Could you check a few things on this drawing? It's one solid part, dimensions in mm from its lowest x, y, z. A direction names the side the tool comes from. Coordinates: 2 decimals unless noted, no trailing zeros. Loops run counter-clockwise (first coordinate to the right, second up) from the corner with the lowest first, then second, coordinate; pieces in that order, holes last.
1) For the marked faces 4 and 5, which set-ups out of +Z, -Z, +X, -X, +Y, -Y let a thin tool reach every point of the face, with its end or its side?
2) Imagine slicing it at D-D on z = 17. Please give me the cut outline in (x, y).
3) Thinking about a two-plate mould opening in Y: for the marked faces 1, 2 and 3, which applies, released by +Y, released by -Y, zero draft, split by the parting line, or undercut?
4) Imagine slicing it at C-C on x = 11. Give the number of separate pieces and of enclosed holes in the cut face.
5) Will these pins go through, and if not, where does the flat tip stop? P1, Ø1, axis at x = 33.5, z = 22.5, coming from the -Y side; P2, Ø5, axis at x = 6.35, y = 51.66, coming from the -Z side; P3, Ø4, axis at x = 11.575, z = 9.525, coming from the +Y side; P4, Ø2, axis at x = 6.5, z = 43.5, coming from the +Y side.
6) If I drill on line 1 along Y through (x, z) = (15, 21); line 2 along Z through (x, y) = (53.5, 46.5); line 3 along Y through (x, z) = (6, 60) (1 decimal), over which ranges is the centre line in solid material (lowest first)?
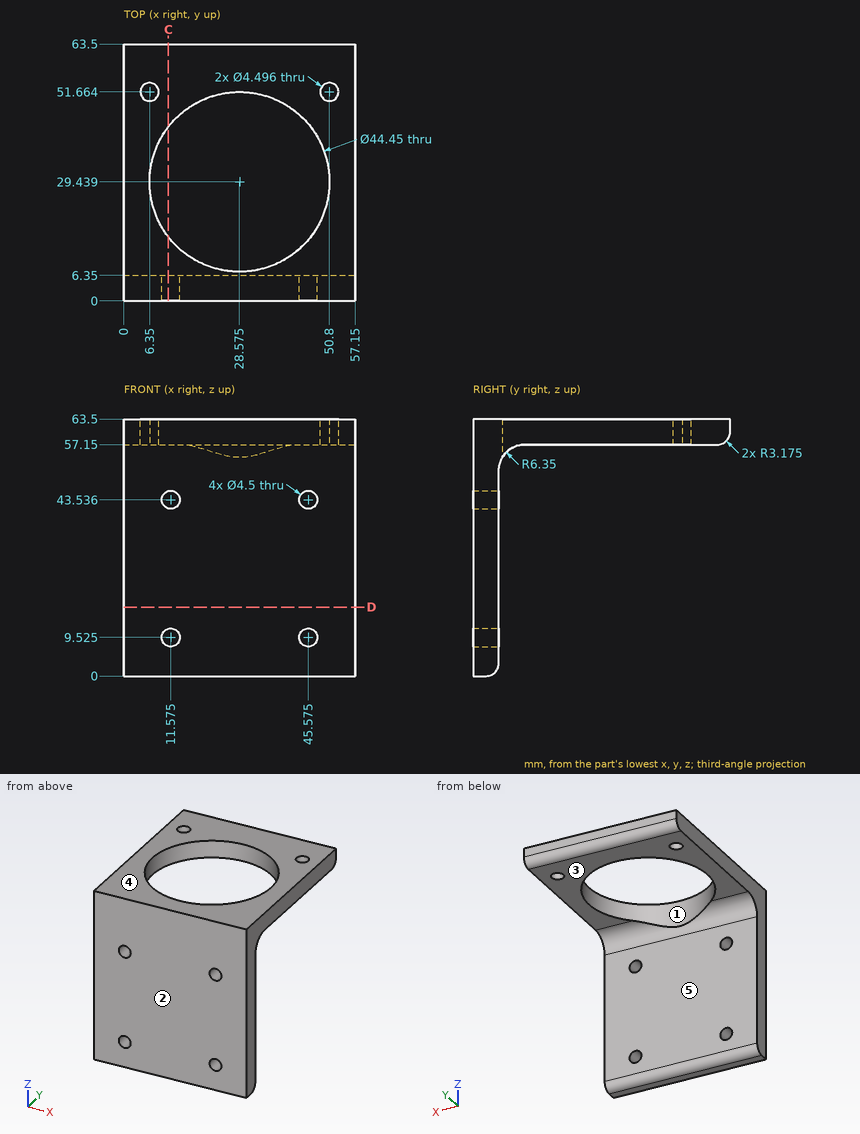
Filled in:
1. face 4: +Z, +X, -X, +Y, -Y
1. face 5: -Z, +X, -X, +Y
2. outline: (0, 0) - (57.15, 0) - (57.15, 6.35) - (0, 6.35) - close
3. face 1: undercut
3. face 2: released by -Y
3. face 3: zero draft
4. separate pieces: 4
4. enclosed holes: 0
5. P1: stops at y = 0
5. P2: stops at z = 57.15
5. P3: passes through
5. P4: stops at y = 6.35
6. line 1: y = 0 to 6.35
6. line 2: z = 57.15 to 63.5
6. line 3: y = 0 to 49.4, 53.9 to 63.5
